Design review of the part built by this model. Coordinates are the model's own, in mm. Give positions to 0.01 mm unless a question says otherwise; leave off trailing zeros. Order: outer loops, then holes, each group sorted by start corner. A loop starts at its lowest first (then second) coordinate and runs counter-clockwise, first axis right, second up. Notation, with made-up numbers: (-25, -16) -> (28, -16) arc R19 cw to (28, 19) -> close; hole circle Ø7 at (19.5, 87.25). An arc over 180 degrees is marked (long way). Return JSON: item names as keys, results as strings.
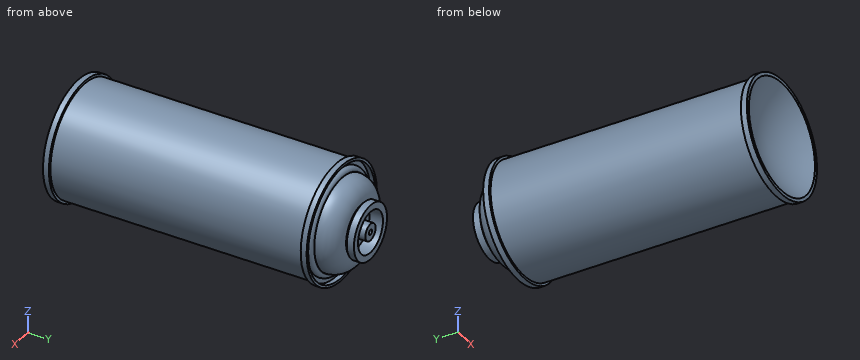
```python
from build123d import *

# Parameters (mm, degrees)
SKETCH1_R           = 33
BOSS_EXTRUDE1_DEPTH = 156
SKETCH3_R           = 34.5
BOSS_EXTRUDE2_DEPTH = 3.5
LPATTERN1_COUNT     = 2
LPATTERN1_PITCH     = 152.5
SKETCH6_R           = 1.5
CUT_EXTRUDE1_DEPTH  = 6
CUT_EXTRUDE2_START  = -3
SKETCH7_R           = 33
SKETCH7_R_2         = 30
CUT_EXTRUDE2_DEPTH  = 3
FILLET1_R           = 2.5


with BuildPart() as part:
    # Sketch1 → Boss-Extrude1 (new body)
    with BuildSketch(Plane(origin=(0, 0, 0), x_dir=(1, 0, 0), z_dir=(0, 1, 0))):
        with Locations(Location((0, 0, 0), (0, 0, 270))):
            Circle(SKETCH1_R)
    extrude(amount=BOSS_EXTRUDE1_DEPTH)

    # Sketch2 → Revolve1 (revolve)
    with BuildSketch(Plane(origin=(0, 0, 0), x_dir=(0, 0, -1), z_dir=(1, 0, 0)), mode=Mode.PRIVATE) as revolve1_sk:
        with BuildLine():
            Line((15.25, 167.75), (15.25, 168.75))
            Line((15.25, 168.75), (16.25, 168.75))
            Line((16.25, 168.75), (16.25, 173))
            Line((16.25, 173), (12.25, 173))
            Line((12.25, 173), (12.25, 165))
            Line((12.25, 165), (5, 165))
            Line((5, 165), (5, 173))
            Line((5, 173), (0, 173))
            Line((0, 173), (0, 156))
            Line((0, 156), (27, 156))
            ThreePointArc((27, 156), (23.558504679, 164.308504679), (15.25, 167.75))
        make_face()
    revolve(revolve1_sk.sketch.rotate(Axis((0, 173, 0), (0, -1, 0)), 180), axis=Axis((0, 173, 0), (0, -1, 0)))

    # Sketch3 → Boss-Extrude2 (add)
    with BuildSketch(Plane(origin=(0, 156, 0), x_dir=(1, 0, 0), z_dir=(0, 1, 0))):
        with Locations(Location((0, 0, 0), (0, 0, 270))):
            Circle(SKETCH3_R)
    boss_extrude2 = extrude(amount=-BOSS_EXTRUDE2_DEPTH)

    # LPattern1: Boss-Extrude2 ×2
    with Locations(*[(0, -i * LPATTERN1_PITCH, 0) for i in range(1, LPATTERN1_COUNT)]):
        add(boss_extrude2)

    # Sketch5 → Cut-Revolve1 (revolve, cut)
    with BuildSketch(Plane.XY, mode=Mode.PRIVATE) as cut_revolve1_sk:
        with BuildLine():
            Line((0, 0), (-32.5, 0))
            ThreePointArc((-32.5, 0), (-17.322312201, 8.904178879), (0, 12))
            Line((0, 12), (0, 0))
        make_face()
    revolve(cut_revolve1_sk.sketch.rotate(Axis((0, 12, 0), (0, -1, 0)), 180), axis=Axis((0, 12, 0), (0, -1, 0)), mode=Mode.SUBTRACT)

    # Sketch6 → Cut-Extrude1 (cut)
    with BuildSketch(Plane(origin=(0, 173, 0), x_dir=(1, 0, 0), z_dir=(0, 1, 0))):
        with Locations(Location((0, 0, 0), (0, 0, 270))):
            Circle(SKETCH6_R)
    extrude(amount=-CUT_EXTRUDE1_DEPTH, mode=Mode.SUBTRACT)

    # Sketch7 → Cut-Extrude2 (cut)
    with BuildSketch(Plane(origin=(0, 156, 0), x_dir=(1, 0, 0), z_dir=(0, 1, 0)).offset(CUT_EXTRUDE2_START)):
        with Locations(Location((0, 0, 0), (0, 0, 270))):
            Circle(SKETCH7_R)
        with Locations(Location((0, 0, 0), (0, 0, 270))):
            Circle(SKETCH7_R_2, mode=Mode.SUBTRACT)
    extrude(amount=CUT_EXTRUDE2_DEPTH, mode=Mode.SUBTRACT)

    # Fillet1
    fillet1_edges = [part.edges().sort_by_distance(p)[0] for p in [
        (0, 156, -30),
    ]]
    fillet(fillet1_edges, radius=FILLET1_R)


solid = part.part
```
Item 1: Wall thickness on L1, parallel to X at y = 170, z = 0; L2, parallel to X at y = 154, z = 0; L3, parallel to X at y = 154.5, z = 0: over which ranges is each line inside the solid? List them lowest first. Write a range as [from, to].
Result set:
{"L1": "x = [-16.25, -12.25], [-5, -1.5], [1.5, 5], [12.25, 16.25]", "L2": "x = [-34.5, -33], [-29.95, 29.95], [33, 34.5]", "L3": "x = [-34.5, -33], [-29.79, 29.79], [33, 34.5]"}
Item 2: For pin 1 (3 mm diameter, centred on y = 119.5, z = 26, fed in from +X); pin 2 (1 mm diameter, centred on y = 109.5, z = 1, fed in from -X); pin 3 (4 mm diameter, centred on y = 126, z = 11, fed in from -X); pin 4 (12 mm diameter, centred on x = 3, z = 6, fed in from +Y), all flat-tipped, find the tip position at first contact; note any pin that passes through.
Result set:
{"pin 1": "stops at x = 22.11", "pin 2": "stops at x = -33", "pin 3": "stops at x = -31.75", "pin 4": "stops at y = 173"}
Item 3: Add section A-A (y = 54.5). Give the boundary of the cut face in (x, z).
Result set:
{"outline": "circle Ø66 at (0, 0)"}
